Part model, mm, in its own coordinate system. A direction names the side the tool comes from. Round coordinates to 2 decimals unless told otherwise and drop trailing zeros. Write each loop counter-clockwise with the first axis right and the second up, starting at its lowest first coordinate (ties: lowest second). Pieces come first, ordered by that corner, then holes.
1) Which spindle directions (+Z, -Z, +X, -X, +Y, -Y) get a long thin tool onto all of the face, cutting with end or side? Do faces 5 (the cylindrical face through (0.651, 14.957, 2.662)), 6 (the flat face through (46, 56, 5)), 7 (the flat face through (2, 21, 0)), 8 (the flat face through (70, 26, 5)). Say none if no direction does.
2) Flat gauge pins, fed straight in: pin 1 (11.5 mm diameter, centred on x = -58, y = 10, fed in from -Z); pin 2 (3.5 mm diameter, centred on x = 58, y = 47, fed in from -Z); pin 3 (1.1 mm diameter, centred on y = 61.5, z = 4, fed in from -X); pin 4 (6 mm diameter, centred on x = 58, y = 47, fed in from -Z). Where does each tip first touch, or does it go through?
3) Saw through at B-B on x = 0. Write the cut outline in (y, z), and give its area (3 significant figures).
4) Saw through at C-C on z = 8. Count the separate pieces of the cut face and the enclosed holes in it, and give its area (3 significant figures).
5) Pull direction X, two halves, no side cores. Call faces 1 (the cylindrical face through (-0.358, 12.727, 7.732)), 2 (the flat face through (-35, 66, 5)), 3 (the cylindrical face through (-57.349, 51.957, 2.662)), 4 (the cylindrical face through (74.684, 67.6, 4.93)): +X half, -X half, draft (parallel to the pull), parting line (faces both ways), or undercut.
6) Drill centre lines: L1, parallel to Y at x = -23.57, z = 3; L2, parallel to Y at x = -4, z = 5; L3, parallel to X at y = 63, z = 5.25. Where is each one in solid material? Low to high.
7) Saw through at D-D on x = -23.57. Write the cut outline in (y, z).
8) Saw through at A-A on y = 10. Write the cut outline in (x, z), and give its area (3 significant figures).
```python
from build123d import *

# Parameters (mm, degrees)
EXTRUDE1_DEPTH                                      = 10
M5_TAPPED_HOLE1_D                                   = 4.2
CUT_EXTRUDE1_REACH                                  = 12
SKETCH4_R                                           = 21
CHAMFER1_SIZE                                       = 3
CBORE_FOR_M5_HEX_SOCKET_HEAD_CAP_SCREW1_D           = 5.5
CBORE_FOR_M5_HEX_SOCKET_HEAD_CAP_SCREW1_CBORE_D     = 10
CBORE_FOR_M5_HEX_SOCKET_HEAD_CAP_SCREW1_CBORE_DEPTH = 5.4
EXTRUDE2_DEPTH                                      = 10
FILLET3_R                                           = 10
FILLET4_R                                           = 5
M12X1_0_TAPPED_HOLE2_D                              = 11
M12X1_0_TAPPED_HOLE1_D                              = 11


with BuildPart() as part:
    # Sketch1 → Extrude1 (new body)
    with BuildSketch(Plane.XY):
        Polygon((35, 56), (70, 56), (70, 0), (-70, 0), (-70, 56), (-35, 56), (-35, 75), (35, 75), align=None)
    extrude(amount=EXTRUDE1_DEPTH)

    # M5 Tapped Hole1 (through all)
    with Locations(Plane(origin=(0, 0, 0), x_dir=(-1, 0, 0), z_dir=(0, 0, -1))):
        with Locations((-23.57, 68.57), (23.57, 68.57), (-23.57, 21.43), (23.57, 21.43)):
            Hole(M5_TAPPED_HOLE1_D / 2)

    # Sketch4 → Cut-Extrude1 (cut, up to next)
    with BuildSketch(Plane.XY.offset(10), mode=Mode.PRIVATE) as cut_extrude1_sk1:
        with Locations((0, 45)):
            Circle(SKETCH4_R)
    cut_extrude1_tool1 = extrude(cut_extrude1_sk1.sketch, amount=-CUT_EXTRUDE1_REACH, mode=Mode.PRIVATE) & part.part
    add(cut_extrude1_tool1.solids().sort_by_distance((0, 45, 10))[0], mode=Mode.SUBTRACT)

    # Chamfer1
    chamfer1_edges = [part.edges().sort_by_distance(p)[0] for p in [
        (-35, 75, 5),
        (35, 75, 5),
    ]]
    chamfer(chamfer1_edges, length=CHAMFER1_SIZE)

    # CBORE for M5 Hex Socket Head Cap Screw1 (through all)
    with Locations(Plane(origin=(0, 0, 0), x_dir=(-1, 0, 0), z_dir=(0, 0, -1))):
        with Locations((-58, 10), (0, 10), (58, 10), (58, 47), (-58, 47)):
            CounterBoreHole(CBORE_FOR_M5_HEX_SOCKET_HEAD_CAP_SCREW1_D / 2, CBORE_FOR_M5_HEX_SOCKET_HEAD_CAP_SCREW1_CBORE_D / 2, CBORE_FOR_M5_HEX_SOCKET_HEAD_CAP_SCREW1_CBORE_DEPTH)

    # Sketch7 → Extrude2 (add)
    with BuildSketch(Plane(origin=(0, 0, 0), x_dir=(-1, 0, 0), z_dir=(0, 0, -1))):
        with BuildLine():
            Line((-66.341582795, 73.222893867), (-56.19763933, 73.222893867))
            Line((-56.19763933, 73.222893867), (-56.19763933, 56))
            Line((-56.19763933, 56), (-70, 56))
            ThreePointArc((-70, 56), (-75.145162885, 66.092914615), (-66.341582795, 73.222893867))
        make_face()
    extrude(amount=-EXTRUDE2_DEPTH)

    # Fillet3
    fillet3_edges = [part.edges().sort_by_distance(p)[0] for p in [
        (56.19763933, 73.222893867, 5),
        (70, 56, 5),
    ]]
    fillet(fillet3_edges, radius=FILLET3_R)

    # Fillet4
    fillet4_edges = [part.edges().sort_by_distance(p)[0] for p in [
        (56.19763933, 56, 5),
        (-35, 56, 5),
        (35, 56, 5),
    ]]
    fillet(fillet4_edges, radius=FILLET4_R)

    # M12x1.0 Tapped Hole2 (through all)
    with Locations(Plane(origin=(0, 0, 0), x_dir=(-1, 0, 0), z_dir=(0, 0, -1))):
        with Locations((-66.341582795, 64.222893867)):
            Hole(M12X1_0_TAPPED_HOLE2_D / 2)

    # M12x1.0 Tapped Hole1 (through all)
    with Locations(Plane(origin=(0, 0, 0), x_dir=(-1, 0, 0), z_dir=(0, 0, -1))):
        with Locations((-66.341582795, 64.222893867)):
            Hole(M12X1_0_TAPPED_HOLE1_D / 2)


solid = part.part
```
Completed:
1. face 5: -Z
1. face 6: +Z, -Z, +Y
1. face 7: -Z, +X, -X, +Y, -Y
1. face 8: +Z, -Z, +X, -Y
2. pin 1: stops at z = 0
2. pin 2: passes through
2. pin 3: stops at x = -35
2. pin 4: stops at z = 5.4
3. outline: (0, 0) - (5, 0) - (5, 5.4) - (7.25, 5.4) - (7.25, 10) - (0, 10) - close; (12.75, 5.4) - (15, 5.4) - (15, 0) - (24, 0) - (24, 10) - (12.75, 10) - close; (66, 0) - (75, 0) - (75, 10) - (66, 10) - close
3. area: 251 mm2
4. separate pieces: 1
4. enclosed holes: 11
4. area: 7,800 mm2
5. face 1: undercut
5. face 2: -X half
5. face 3: undercut
5. face 4: +X half
6. L1: y = 0 to 19.33, 23.53 to 66.47, 70.67 to 75
6. L2: y = 0 to 7, 13 to 24.38, 65.62 to 75
6. L3: x = -35 to -10.82, 10.82 to 35, 56.2 to 60.98, 71.7 to 75.26
7. outline: (0, 0) - (19.33, 0) - (19.33, 10) - (0, 10) - close; (23.53, 0) - (66.47, 0) - (66.47, 10) - (23.53, 10) - close; (70.67, 0) - (75, 0) - (75, 10) - (70.67, 10) - close
8. outline: (-70, 0) - (-63, 0) - (-63, 5.4) - (-60.75, 5.4) - (-60.75, 10) - (-70, 10) - close; (-55.25, 5.4) - (-53, 5.4) - (-53, 0) - (-5, 0) - (-5, 5.4) - (-2.75, 5.4) - (-2.75, 10) - (-55.25, 10) - close; (2.75, 5.4) - (5, 5.4) - (5, 0) - (53, 0) - (53, 5.4) - (55.25, 5.4) - (55.25, 10) - (2.75, 10) - close; (60.75, 5.4) - (63, 5.4) - (63, 0) - (70, 0) - (70, 10) - (60.75, 10) - close
8. area: 1,160 mm2
